The drawing under review shows one solid part. Ordinate dimensions are in mm from its lowest x, y, z. Give positions to 0.01 mm unless a question says otherwise; leave off trailing zeros. Order: outer loops, then holes, each group sorted by start corner. A loop starts at its lowest first (then second) coordinate and runs counter-clockwise, first axis right, second up. Notation, with made-up numbers: (0, 67.5) -> (39, 67.5) arc R35 ccw to (39, 101.5) -> close; hole circle Ø8 at (-23, 22). An arc over 180 degrees is marked (long way). One line per item, written item: value.
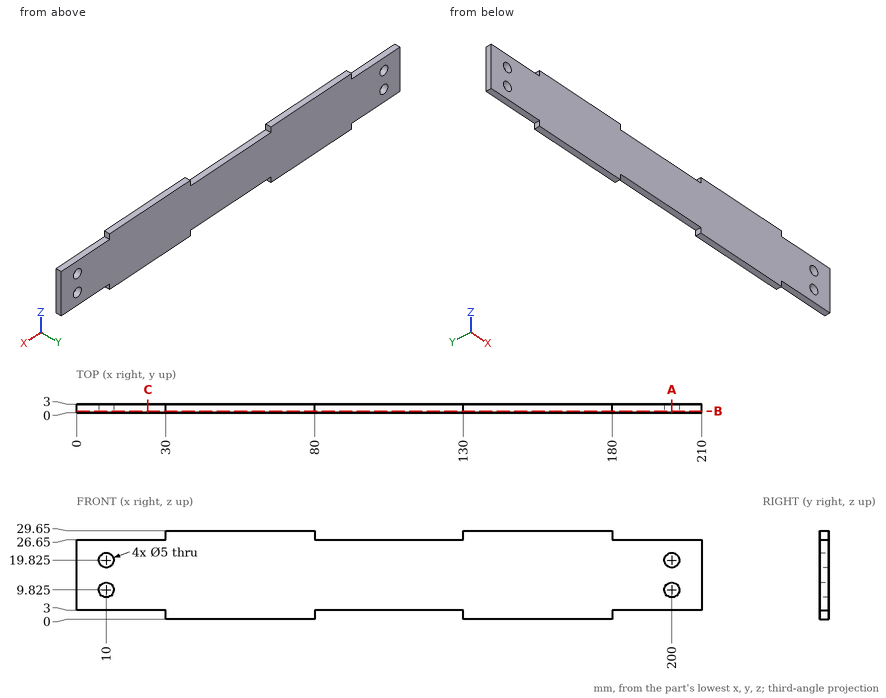
Item 1: Add section B-B on y = 0.6. Give the boundary of the cut face in (x, z) (3 decimals).
Returned:
outline: (0, 3) -> (30, 3) -> (30, 0) -> (80, 0) -> (80, 3) -> (130, 3) -> (130, 0) -> (180, 0) -> (180, 3) -> (210, 3) -> (210, 26.65) -> (180, 26.65) -> (180, 29.65) -> (130, 29.65) -> (130, 26.65) -> (80, 26.65) -> (80, 29.65) -> (30, 29.65) -> (30, 26.65) -> (0, 26.65) -> close; hole circle Ø5 at (10, 9.825); hole circle Ø5 at (10, 19.825); hole circle Ø5 at (200, 9.825); hole circle Ø5 at (200, 19.825)
Item 2: To check wall thickness, follow line 1 along Z through (x, y) = (200, 1.15) (3 decimals); line 2 along X through (y, z) = (1.45, 19.75); line 3 along X through (y, z) = (0.8, 2). State the ranges of each line that lie inside material, in increasing order. Write a range as from..to.
Returned:
line 1: 3..7.325, 12.325..17.325, 22.325..26.65
line 2: 0..7.5, 12.5..197.5, 202.5..210
line 3: 30..80, 130..180
Item 3: Add section A-A on x = 200. Give the boundary of the cut face in (y, z) (3 decimals), plus the area to 4 significant figures.
Returned:
outline: (0, 3) -> (3, 3) -> (3, 7.325) -> (0, 7.325) -> close; (0, 12.325) -> (3, 12.325) -> (3, 17.325) -> (0, 17.325) -> close; (0, 22.325) -> (3, 22.325) -> (3, 26.65) -> (0, 26.65) -> close
area: 40.95 mm²
Item 4: Add section C-C on x = 24. Give the boundary of the cut face in (y, z), plus the area to 4 significant figures.
Returned:
outline: (0, 3) -> (3, 3) -> (3, 26.65) -> (0, 26.65) -> close
area: 70.95 mm²
Item 5: Clearance check with flat-ended pins moving along their axes: P1, Ø1.5, axis at x = 192.5, y = 1, coming from the +Z side; P2, Ø12, axis at x = 137, z = 16.5, coming from the -Y side; P3, Ø0.9, axis at y = 1, z = 27.5, coming from the +X side; P4, Ø1.5, axis at y = 2, z = 28.5, coming from the -X side. State where each tip first meets the part, or that it passes through.
Returned:
P1: z = 26.65
P2: y = 0
P3: x = 180
P4: x = 30
